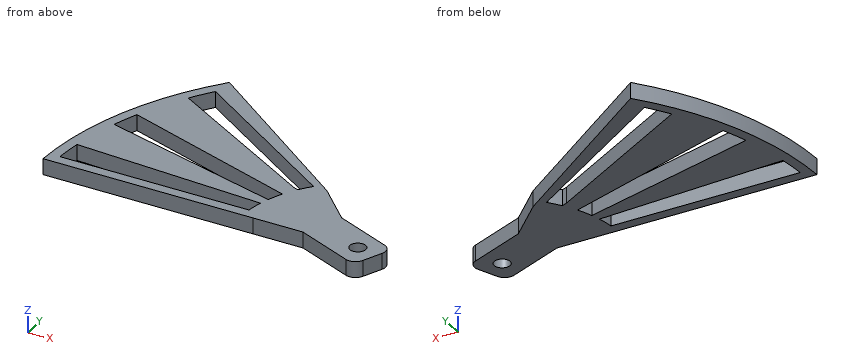
from build123d import *

# Parameters (mm, degrees)
BOSS_EXTRUDE2_DEPTH = 3
CUT_EXTRUDE1_DEPTH  = 4
SKETCH1_8_R         = 1.5
BOSS_EXTRUDE5_DEPTH = 3
FILLET1_R           = 2


with BuildPart() as part:
    # Sketch1 → Boss-Extrude2 (new body)
    with BuildSketch(Plane.XY):
        with BuildLine():
            Line((-19.985447982, 0.762803358), (-59.956343946, 2.288410074))
            ThreePointArc((-59.956343946, 2.288410074), (-55.730717245, 22.228071336), (-45.073672701, 39.602576043))
            Line((-45.073672701, 39.602576043), (-13.592462366, 14.67122922))
            ThreePointArc((-13.592462366, 14.67122922), (-18.172234131, 8.352838241), (-19.985447982, 0.762803358))
        make_face()
    extrude(amount=BOSS_EXTRUDE2_DEPTH)

    # Sketch1_5 → Cut-Extrude1 (cut, through all)
    with BuildSketch(Plane.XY):
        with BuildLine():
            ThreePointArc((-21.816681027, 2.834154011), (-21.572673921, 4.315059664), (-21.2282638, 5.775882272))
            Line((-21.2282638, 5.775882272), (-57.269563461, 9.175897829))
            ThreePointArc((-57.269563461, 9.175897829), (-57.611850796, 6.698854216), (-57.847050894, 4.209358967))
            Line((-57.847050894, 4.209358967), (-21.816681027, 2.834154011))
        make_face()
        with BuildLine():
            Line((-18.974652115, 13.123988942), (-17.985708937, 12.669422798))
            ThreePointArc((-17.985708937, 12.669422798), (-17.201666988, 13.715052053), (-16.356919422, 14.712280144))
            Line((-16.356919422, 14.712280144), (-16.19149009, 14.894148135))
            Line((-16.19149009, 14.894148135), (-45.633154018, 35.799654388))
            ThreePointArc((-45.633154018, 35.799654388), (-47.133831778, 33.799436415), (-48.546898537, 31.736393028))
            Line((-48.546898537, 31.736393028), (-18.974652115, 13.123988942))
        make_face()
        with BuildLine():
            Line((-55.106686022, 18.090139737), (-20.700540486, 7.449001516))
            ThreePointArc((-20.700540486, 7.449001516), (-20.144482043, 8.843067523), (-19.494667642, 10.19597634))
            Line((-19.494667642, 10.19597634), (-53.343874365, 22.769081398))
            ThreePointArc((-53.343874365, 22.769081398), (-54.275723264, 20.448615214), (-55.106686022, 18.090139737))
        make_face()
    extrude(amount=CUT_EXTRUDE1_DEPTH, mode=Mode.SUBTRACT)

    # Sketch1_8 → Boss-Extrude5 (add)
    with BuildSketch(Plane.XY):
        with BuildLine():
            Line((-7.103763171, 7.667553899), (-13.592462366, 14.67122922))
            ThreePointArc((-13.592462366, 14.67122922), (-18.172234131, 8.352838241), (-19.985447982, 0.762803358))
            Line((-19.985447982, 0.762803358), (-10.444898468, 0.398660247))
            Line((-10.444898468, 0.398660247), (1.963879178, -5.305014474))
            Line((1.963879178, -5.305014474), (5.305014474, 1.963879178))
            Line((5.305014474, 1.963879178), (-7.103763171, 7.667553899))
        make_face()
        Circle(SKETCH1_8_R, mode=Mode.SUBTRACT)
    extrude(amount=BOSS_EXTRUDE5_DEPTH)

    # Fillet1
    fillet1_edges = [part.edges().sort_by_distance(p)[0] for p in [
        (1.963879178, -5.305014474, 1.5),
        (5.305014474, 1.963879178, 1.5),
    ]]
    fillet(fillet1_edges, radius=FILLET1_R)


solid = part.part
The model under review builds one solid part; all positions refer to its coordinate system, in mm. Round coordinates to 2 decimals unless told otherwise and drop trailing zeros. Loops run counter-clockwise (first coordinate to the right, second up) from the corner with the lowest first, then second, coordinate; pieces in that order, holes last. Notation, with made-up numbers: (-34, -23) - (-17, -23) arc R17 cw to (-17, 2) - close; hole circle Ø4 at (17.5, 29.25). An arc over 180 degrees is marked (long way). Use CSV: the item, a comma, the result in double quotes.
(1) Take a section at B-B, the plane y = 11. Give the boundary of the cut face in (x, z), plus the area to 3 significant figures.
Working result:
outline,"(-58.98, 0) - (-32.18, 0) - (-32.18, 3) - (-58.98, 3) - close; (-21.66, 0) - (-10.19, 0) - (-10.19, 3) - (-21.66, 3) - close"
area,"115 mm^2"
(2) Take a section at A-A, the plane z = 0.75. Give the boundary of the cut face in (x, y), plus the area to 3 significant figures.
Working result:
outline,"(-59.96, 2.29) - (-10.44, 0.4) - (0.15, -4.47) arc R2 ccw to (2.8, -3.49) - (4.47, 0.15) arc R2 ccw to (3.49, 2.8) - (-7.1, 7.67) - (-13.59, 14.67) - (-45.07, 39.6) arc R60 ccw to start; hole (-57.85, 4.21) - (-21.82, 2.83) arc R22 cw to (-21.23, 5.78) - (-57.27, 9.18) arc R58 ccw to start; hole (-55.11, 18.09) - (-20.7, 7.45) arc R22 cw to (-19.49, 10.2) - (-53.34, 22.77) arc R58 ccw to start; hole (-48.55, 31.74) - (-18.97, 13.12) - (-17.99, 12.67) arc R22 cw to (-16.36, 14.71) - (-16.19, 14.89) - (-45.63, 35.8) arc R58 ccw to start; hole circle Ø3 at (0, 0)"
area,"920 mm^2"
(3) Clearance check with a flat-ended pin moving along its axis: P1, Ø5, axis at x = -3.5, y = 11.5, coming from the -Z side. State where the tip first meets the part, or that it passes through.
Working result:
P1,"passes through"
(4) For line 1 (Y direction, x = -51.5, z = 0.5); line 2 (Y direction, x = -45, z = 1.6); line 3 (Y direction, x = -41, z = 2.6), list the stretches that pass through material, from the lowest coordinate up.
Working result:
line 1,"y = 1.97 to 3.97, 8.63 to 16.97, 22.08 to 30.79"
line 2,"y = 1.72 to 3.72, 8.02 to 14.96, 19.67 to 29.5, 35.35 to 39.54"
line 3,"y = 1.56 to 3.57, 7.64 to 13.73, 18.18 to 26.99, 32.51 to 36.38"
(5) Take a section at D-D, the plane y = 20. Give the boundary of the cut face in (x, z), plus the area to 3 significant figures.
Working result:
outline,"(-56.57, 0) - (-54.44, 0) - (-54.44, 3) - (-56.57, 3) - close; (-45.89, 0) - (-29.9, 0) - (-29.9, 3) - (-45.89, 3) - close; (-23.38, 0) - (-20.32, 0) - (-20.32, 3) - (-23.38, 3) - close"
area,"63.5 mm^2"
(6) Take a section at C-C, the plane x = -42.5. Give the boundary of the cut face in (y, z).
Working result:
outline,"(1.62, 0) - (3.62, 0) - (3.62, 3) - (1.62, 3) - close; (7.78, 0) - (14.19, 0) - (14.19, 3) - (7.78, 3) - close; (18.74, 0) - (27.93, 0) - (27.93, 3) - (18.74, 3) - close; (33.57, 0) - (37.56, 0) - (37.56, 3) - (33.57, 3) - close"
